For this review, take the finished solid that the model builds, in its own axes (mm). Face numbers are marked on the shaded views. A direction names the side the tool comes from. Give positions to 0.01 mm unless a question says otherwise; leave off trailing zeros. Loops run counter-clockwise (first coordinate to the right, second up) from the corner with the lowest first, then second, coordinate; pieces in that order, holes last.
```python
from build123d import *

# Parameters (mm, degrees)
SFAZOWANIE2_SIZE            = 1
SZKIC2_W                    = 27
SZKIC2_H                    = 0.05
SZKIC3_R                    = 4
DODANIE_WYCI_GNI_CIE1_DEPTH = 5.3
SFAZOWANIE3_SIZE            = 0.5


with BuildPart() as part:
    # Szkic1 → Obrót1 (revolve)
    with BuildSketch(Plane.XY, mode=Mode.PRIVATE) as obr_t1_sk:
        Polygon((0, 4), (33, 4), (33, 6.35), (3, 6.35), (3, 7.75), (0, 7.75), align=None)
    revolve(obr_t1_sk.sketch.rotate(Axis((0, 0, 0), (1, 0, 0)), 90), axis=Axis((0, 0, 0), (1, 0, 0)))

    # Sfazowanie2
    sfazowanie2_edges = [part.edges().sort_by_distance(p)[0] for p in [
        (33, 0, -6.35),
    ]]
    chamfer(sfazowanie2_edges, length=SFAZOWANIE2_SIZE)

    # Szkic2 → Wycięcie-obrót1 (revolve, cut)
    with BuildSketch(Plane.XY, mode=Mode.PRIVATE) as wyci_cie_obr_t1_sk:
        with Locations((16.5, 6.325)):
            Rectangle(SZKIC2_W, SZKIC2_H)
    revolve(wyci_cie_obr_t1_sk.sketch.rotate(Axis((3, 0, 0), (1, 0, 0)), 90), axis=Axis((3, 0, 0), (1, 0, 0)), mode=Mode.SUBTRACT)

    # Szkic3 → Dodanie-wyciągnięcie1 (add)
    with BuildSketch(Plane.ZY):
        Polygon((6.5, -3.75277675), (6.5, 3.75277675), (0, 7.505553499), (-6.5, 3.75277675), (-6.5, -3.75277675), (0, -7.505553499), align=None)
        Circle(SZKIC3_R, mode=Mode.SUBTRACT)
    extrude(amount=DODANIE_WYCI_GNI_CIE1_DEPTH)

    # Szkic4 → Wycięcie-obrót2 (revolve, cut)
    with BuildSketch(Plane(origin=(0, 0, 0), x_dir=(1, 0, 0), z_dir=(0, 1, 0)), mode=Mode.PRIVATE) as wyci_cie_obr_t2_sk:
        Polygon((-5.3, 6.5), (-5.3, 10), (-1.8, 10), align=None)
    revolve(wyci_cie_obr_t2_sk.sketch.rotate(Axis((0, 0, 0), (-1, 0, 0)), 180), axis=Axis((0, 0, 0), (-1, 0, 0)), mode=Mode.SUBTRACT)

    # Sfazowanie3
    sfazowanie3_edges = [part.edges().sort_by_distance(p)[0] for p in [
        (-5.3, 0, -4),
    ]]
    chamfer(sfazowanie3_edges, length=SFAZOWANIE3_SIZE)


solid = part.part
```
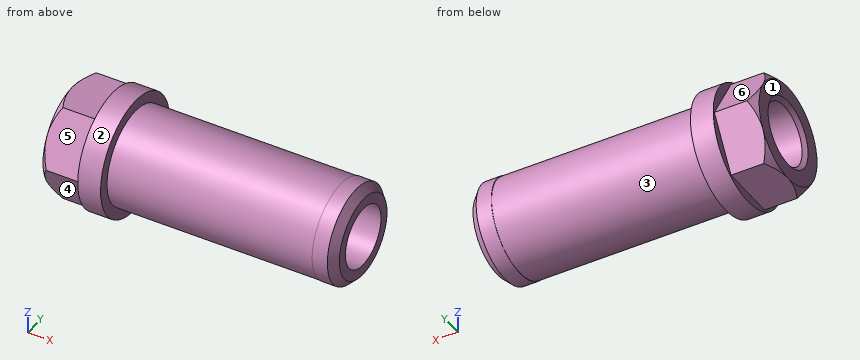
Item 1: Tool access review of the marked faces 4, 5 and 6: name each direction out of +Z, -Z, +X, -X, +Y, -Y from which nothing blocks a thin tool from reaching the whole face with its end or side.
Answer:
face 4: -Z, -X, -Y
face 5: +Z, -X, -Y
face 6: +Z, -X, +Y
Item 2: For L1, parallel to Y at x = 8.5, z = 0; L2, parallel to Z at x = -1.95, y = 0; L3, parallel to Y at x = -1.15, z = 0, list the stretches that pass through material, from the lowest coordinate up.
Answer:
L1: y = -6.3 to -4, 4 to 6.3
L2: z = -6.5 to -4, 4 to 6.5
L3: y = -7.51 to -4, 4 to 7.51
Item 3: The part is to be moulded in two halves that separate along X. For the marked faces 1, 2 and 3, say which applies: released by +X, released by -X, zero draft, split by the parting line, or undercut.
Answer:
face 1: released by -X
face 2: zero draft
face 3: undercut
Item 4: Clearance check with flat-ended pins moving along their axes: pin 1 Ø5 at (x, z) = (26.5, 4) entering from -Y; pin 2 Ø2.5 at (x, y) = (-2.5, 1.5) entering from -Z; pin 3 Ø1.6 at (x, y) = (-1.5, -1.5) entering from +Z. State where each tip first meets the part, or that it passes through.
Answer:
pin 1: stops at y = -6.12
pin 2: stops at z = -6.5
pin 3: stops at z = 6.5
Item 5: Take a section at A-A on x = 19. Give the boundary of the cut face in (y, z), and give its area (3 significant figures).
Answer:
outline: circle Ø12.6 at (0, 0); hole circle Ø8 at (0, 0)
area: 74.4 mm2
